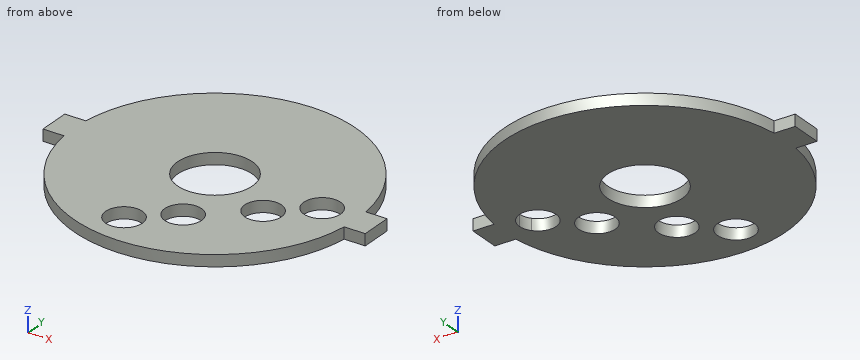
from build123d import *

# Parameters (mm, degrees)
F0_R     = 3.2
F0_R_2   = 6.5
F1_DEPTH = 2


# Not quite as in the source:
# - a feature names something its author has since deleted; it is built from what else it names


with BuildPart() as f1:
    # F0 (on Top) → F1 (new body)
    with BuildSketch(Plane.XY):
        with BuildLine():
            Line((21, 2.75), (24.3451740598, 2.75))
            ThreePointArc((24.3451740598, 2.75), (0, 24.5), (-24.3451740598, 2.75))
            Line((-24.3451740598, 2.75), (-21, 2.75))
            Line((-21, 2.75), (-21, -2.75))
            Line((-21, -2.75), (-24.3451740598, -2.75))
            ThreePointArc((-24.3451740598, -2.75), (0, -24.5), (24.3451740598, -2.75))
            Line((24.3451740598, -2.75), (21, -2.75))
            Line((21, -2.75), (21, -1.9091370521))
            ThreePointArc((21, -1.9091370521), (15.3353042136, 0.1317634061), (21, 2.1726638643))
            Line((21, 2.1726638643), (21, 2.75))
        make_face()
        with Locations((-3.267275868, -18.2230044156)):
            Circle(F0_R, mode=Mode.SUBTRACT)
        with Locations((3.235248016, -12.7487754162)):
            Circle(F0_R, mode=Mode.SUBTRACT)
        Circle(F0_R_2, mode=Mode.SUBTRACT)
        with Locations((12.0327803296, -5.3424655934)):
            Circle(F0_R, mode=Mode.SUBTRACT)
        with BuildLine():
            Line((-21, 2.75), (-24.3451740598, 2.75))
            ThreePointArc((-24.3451740598, 2.75), (-24.5, 0), (-24.3451740598, -2.75))
            Line((-24.3451740598, -2.75), (-21, -2.75))
            Line((-21, -2.75), (-21, 2.75))
        make_face()
        with BuildLine():
            ThreePointArc((-24.3451740598, -2.75), (-24.5, 0), (-24.3451740598, 2.75))
            Line((-24.3451740598, 2.75), (-28, 2.75))
            Line((-28, 2.75), (-28, -2.75))
            Line((-28, -2.75), (-24.3451740598, -2.75))
        make_face()
        with BuildLine():
            ThreePointArc((24.3451740598, -2.75), (24.4612628912, -1.3771774642), (24.5, 0))
            ThreePointArc((24.5, 0), (24.4612628912, 1.3771774642), (24.3451740598, 2.75))
            Line((24.3451740598, 2.75), (21, 2.75))
            Line((21, 2.75), (21, 2.1726638643))
            ThreePointArc((21, 2.1726638643), (21.5458711466, 1.2164231415), (21.7353042136, 0.1317634061))
            ThreePointArc((21.7353042136, 0.1317634061), (21.5458711466, -0.9528963294), (21, -1.9091370521))
            Line((21, -1.9091370521), (21, -2.75))
            Line((21, -2.75), (24.3451740598, -2.75))
        make_face()
        with BuildLine():
            ThreePointArc((24.3451740598, 2.75), (24.4612628912, 1.3771774642), (24.5, 0))
            ThreePointArc((24.5, 0), (24.4612628912, -1.3771774642), (24.3451740598, -2.75))
            Line((24.3451740598, -2.75), (28, -2.75))
            Line((28, -2.75), (28, 2.75))
            Line((28, 2.75), (24.3451740598, 2.75))
        make_face()
    extrude(amount=F1_DEPTH)


solid = f1.part
Source: CAD feature listing. Evaluate the final solid. Frame: model axes, mm. Round coordinates to 2 decimals unless told otherwise and drop trailing zeros. Order: outer loops, then holes, each group sorted by start corner. A loop starts at its lowest first (then second) coordinate and runs counter-clockwise, first axis right, second up. Notation, with made-up numbers: (2.25, 79.25) - (20.25, 79.25) arc R14 cw to (20.25, 97.25) - close; hole circle Ø11 at (14.25, 44). An arc over 180 degrees is marked (long way). Use a Markdown table: item, result. Add a question column.
1. Section query A-A (y = -17.5). Return the cut outline in (x, z).
2. First-contact query: pin 1 (1 mm diameter, centred on x = 26.5, z = 0.5, fed in from +Y); pin 2 (6 mm diameter, centred on x = 3.24, y = -12.75, fed in from +Z); pin 3 (1 mm diameter, centred on x = 26, z = 0.5, fed in from -Y); pin 4 (1 mm diameter, centred on y = -5, z = 0.5, fed in from +X). Flat tips, straight axial feed; report the tip coordinate or a pass-through.
3. Section query D-D (y = 15). Return the cut outline in (x, z).
4. Line query: probe 1 along Y at (x, z) = (-5.5, 0.55); probe 2 along X at (y, z) = (-4, 1.7); probe 3 along Y at (x, z) = (-5, 1.6). Output: solid intervals per line, ascending.
5. Section query C-C (x = -20.5). Return the cut outline in (y, z).
6. Section query B-B (z = 0.65). Return the cut outline in (x, y), then the cut area to 3 significant figures.
Derived:
| question | item | result |
|---|---|---|
| 1 | outline | (-17.15, 0) - (-6.38, 0) - (-6.38, 2) - (-17.15, 2) - close; (-0.15, 0) - (17.15, 0) - (17.15, 2) - (-0.15, 2) - close |
| 2 | pin 1 | y = 2.75 |
| 2 | pin 2 | through |
| 2 | pin 3 | y = -2.75 |
| 2 | pin 4 | x = 24.08 |
| 3 | outline | (-19.37, 0) - (19.37, 0) - (19.37, 2) - (-19.37, 2) - close |
| 4 | probe 1 | -23.87 to -20.52, -15.93 to -3.46, 3.46 to 23.87 |
| 4 | probe 2 | -24.17 to -5.12, 5.12 to 9.13, 14.94 to 24.17 |
| 4 | probe 3 | -23.98 to -20.91, -15.53 to -4.15, 4.15 to 23.98 |
| 5 | outline | (-13.42, 0) - (13.42, 0) - (13.42, 2) - (-13.42, 2) - close |
| 6 | outline | (-28, -2.75) - (-24.35, -2.75) arc R24.5 ccw to (24.35, -2.75) - (28, -2.75) - (28, 2.75) - (24.35, 2.75) arc R24.5 ccw to (-24.35, 2.75) - (-28, 2.75) - close; hole circle Ø13 at (0, 0); hole circle Ø6.4 at (-3.27, -18.22); hole circle Ø6.4 at (3.24, -12.75); hole circle Ø6.4 at (12.03, -5.34); hole circle Ø6.4 at (18.54, 0.13) |
| 6 | area | 1,660 mm2 |
